For this review, take the finished solid that the model builds, in its own axes (mm). A direction names the side the tool comes from. Give positions to 0.01 mm unless a question says otherwise; leave off trailing zeros. Loops run counter-clockwise (first coordinate to the right, second up) from the corner with the lowest first, then second, coordinate; pieces in that order, holes last. Notation, with made-up numbers: (72, -32) -> (104, -32) arc R3 cw to (104, -27) -> close; hole circle Ø4 at (42.5, 55.5). An arc over 180 degrees is marked (long way). One line per question, with ' | ' between items. Start each with the question number.
(1) Consider section A-A (z = 49). Write out the cut boundary in (x, y), and give its area (3 significant figures).
(2) Wall thickness on probe 1 along Z at (x, y) = (-33.5, -11); probe 2 along Y at (x, z) = (-28.5, 46); probe 3 along Z at (x, y) = (-55, 0): over which ranges is each line inside the solid? List them lowest first.
(3) Consider section B-B (z = 30). Write out the cut boundary in (x, y), and give its area (3 significant figures).
(4) Tool access review of faces 1 (the flat face through (-16.684, 8, 48)), 2 (the flat face through (-29, 19.449, 48)), 3 (the flat face through (-40.282, 8, 48)), 4 (the flat face through (-41, 8, 44.45)), 5 (the cylindrical face through (-38.754, -2.699, 48.313)): name each direction out of +Z, -Z, +X, -X, +Y, -Y from which nothing blocks a thin tool from reaching the whole face with its end or side.
(5) Insertion check: P1, Ø6, axis at x = -27, z = 48.5, coming from the +Y side; P2, Ø3, axis at x = -35, z = 18.5, coming from the -Y side; P3, Ø5, axis at x = -14, z = 13, coming from the +Y side; P4, Ø16, axis at x = -41, y = 12.5, coming from the +Z side. Each pin has a flat end and moves straight along its axis. Give the tip position at first contact, or say it passes through.
from build123d import *

# Parameters (mm, degrees)
F0_R     = 31.75
F1_DEPTH = 44.45
F2_W     = 23.59742
F2_H     = 23.59742
F3_DEPTH = 12.7
F4_R     = 5.08


with BuildPart() as f1:
    # F0 (on Top) → F1 (new body)
    with BuildSketch(Plane.XY):
        with Locations((-28.482823, 7.650726)):
            Circle(F0_R)
    extrude(amount=F1_DEPTH)

    # F2 (on face) → F3 (join)
    with BuildSketch(Plane.XY.offset(44.45)):
        with Locations((-28.482823, 7.650726)):
            Rectangle(F2_W, F2_H)
    extrude(amount=F3_DEPTH)

    # F4
    f4_edges = [f1.edges().sort_by_distance(p)[0] for p in [
        (-60.232823, 7.650726, 44.45),
        (-60.232823, 7.650726, 0),
        (-16.684113, 7.650726, 57.15),
        (-28.482823, -4.147984, 57.15),
        (-40.281533, 7.650726, 57.15),
        (-28.482823, 19.449436, 57.15),
        (-16.684113, -4.147984, 50.8),
        (-40.281533, -4.147984, 50.8),
        (-16.684113, 19.449436, 50.8),
        (-40.281533, 19.449436, 50.8),
    ]]
    fillet(f4_edges, radius=F4_R)


solid = f1.part
A:
1) outline: (-40.28, 0.93) arc R5.08 ccw to (-35.2, -4.15) -> (-21.76, -4.15) arc R5.08 ccw to (-16.68, 0.93) -> (-16.68, 14.37) arc R5.08 ccw to (-21.76, 19.45) -> (-35.2, 19.45) arc R5.08 ccw to (-40.28, 14.37) -> close | area: 535 mm^2
2) probe 1: z = 0 to 44.45 | probe 2: y = -4.15 to 19.45 | probe 3: z = 0.09 to 44.36
3) outline: circle Ø63.5 at (-28.48, 7.65) | area: 3,170 mm^2
4) face 1: +Z, +X, +Y, -Y | face 2: +Z, +X, -X, +Y | face 3: +Z, -X, +Y, -Y | face 4: +Z | face 5: +Z, -X, -Y
5) P1: stops at y = 19.45 | P2: stops at y = -23.7 | P3: stops at y = 37.05 | P4: stops at z = 57.15
